Geometry check sheet. Reference: the model listing, model coordinates, mm. A direction names the side the tool comes from. Coordinates: 2 decimals unless noted, no trailing zeros. Write each loop counter-clockwise with the first axis right and the second up, starting at its lowest first coordinate (ties: lowest second). Pieces come first, ordered by that corner, then holes. Notation, with made-up numbers: (6, 36.25) -> (55, 36.25) arc R16 ccw to (55, 46.25) -> close; hole circle Ø8 at (39.25, 38.5). An arc over 180 degrees is marked (long way). One line per question, with ' | ' between items.
```python
from build123d import *

# Parameters (mm, degrees)
SKETCH1_R           = 5
BOSS_EXTRUDE1_DEPTH = 5
FILLET1_R           = 5
SKETCH2_R           = 0.6
CUT_EXTRUDE1_DEPTH  = 5
SKETCH3_R           = 0.6
CUT_EXTRUDE2_DEPTH  = 2.5
BOSS_EXTRUDE7_REACH = 72.882
BOSS_EXTRUDE8_DEPTH = 35
SKETCH13_R          = 1
SKETCH13_W          = 14
SKETCH13_H          = 24
CUT_EXTRUDE3_DEPTH  = 82.57977968
SKETCH14_W          = 10
SKETCH14_H          = 35
BOSS_EXTRUDE9_DEPTH = 5
SKETCH15_R          = 1.25
CUT_EXTRUDE4_DEPTH  = 5
SKETCH16_R          = 1.25
CUT_EXTRUDE5_DEPTH  = 96.984672029
FILLET2_R           = 5


with BuildPart() as part:
    # Sketch1 → Boss-Extrude1 (new body)
    with BuildSketch(Plane.XY):
        with BuildLine():
            ThreePointArc((0, 10), (-10, 0), (0, -10))
            ThreePointArc((0, -10), (30, -5.393920142), (60, -10))
            ThreePointArc((60, -10), (70, 0), (60, 10))
            ThreePointArc((60, 10), (30, 5.393920142), (0, 10))
        make_face()
        Circle(SKETCH1_R, mode=Mode.SUBTRACT)
        with Locations((60, 0)):
            Circle(SKETCH1_R, mode=Mode.SUBTRACT)
    extrude(amount=BOSS_EXTRUDE1_DEPTH)

    # Fillet1
    fillet1_edges = [part.edges().sort_by_distance(p)[0] for p in [
        (60, 10, 2.5),
        (60, -10, 2.5),
        (0, -10, 2.5),
        (0, 10, 2.5),
    ]]
    fillet(fillet1_edges, radius=FILLET1_R)

    # Sketch2 → Cut-Extrude1 (cut)
    with BuildSketch(Plane(origin=(0, 0, 0), x_dir=(-1, 0, 0), z_dir=(0, 0, -1))):
        with Locations((-4.45, 0)):
            Circle(SKETCH2_R)
        with Locations((-6.45, 0)):
            Circle(SKETCH2_R)
        with Locations((-8.45, 0)):
            Circle(SKETCH2_R)
        with Locations((-10.45, 0)):
            Circle(SKETCH2_R)
        with Locations((-12.45, 0)):
            Circle(SKETCH2_R)
        with Locations((-14.45, 0)):
            Circle(SKETCH2_R)
    cut_extrude1 = extrude(amount=-CUT_EXTRUDE1_DEPTH, mode=Mode.SUBTRACT)

    # Sketch3 → Cut-Extrude2 (cut)
    with BuildSketch(Plane(origin=(0, 0, 0), x_dir=(-1, 0, 0), z_dir=(0, 0, -1))):
        with BuildLine():
            Line((-15.012283737, -2.435946838), (-1.124567474, -4.871893677))
            ThreePointArc((-1.124567474, -4.871893677), (-3.832599709, -3.211102532), (-4.993539326, -0.254096441))
            ThreePointArc((-4.993539326, -0.254096441), (-5.05, 0), (-4.993539326, 0.254096441))
            ThreePointArc((-4.993539326, 0.254096441), (-3.746221254, 3.311468906), (-0.865051903, 4.924600005))
            Line((-0.865051903, 4.924600005), (-14.882525952, 2.462300002))
            ThreePointArc((-14.882525952, 2.462300002), (-16.949123268, 0.066203422), (-15.012283737, -2.435946838))
        make_face()
        with Locations((-12.45, 0)):
            Circle(SKETCH3_R, mode=Mode.SUBTRACT)
        with Locations((-6.45, 0)):
            Circle(SKETCH3_R, mode=Mode.SUBTRACT)
        with Locations((-8.45, 0)):
            Circle(SKETCH3_R, mode=Mode.SUBTRACT)
        with Locations((-10.45, 0)):
            Circle(SKETCH3_R, mode=Mode.SUBTRACT)
        with Locations((-14.45, 0)):
            Circle(SKETCH3_R, mode=Mode.SUBTRACT)
    cut_extrude2 = extrude(amount=-CUT_EXTRUDE2_DEPTH, mode=Mode.SUBTRACT)

    # Mirror2: Cut-Extrude1, Cut-Extrude2 across plane
    add(cut_extrude1.mirror(Plane(origin=(30, 0, 0), x_dir=(0, 0, 1), z_dir=(1, 0, 0))), mode=Mode.SUBTRACT)
    add(cut_extrude2.mirror(Plane(origin=(30, 0, 0), x_dir=(0, 0, 1), z_dir=(1, 0, 0))), mode=Mode.SUBTRACT)

    # Boss-Extrude7: up to this face of the body (flat: up to its plane)
    boss_extrude7_end = Plane(part.part.faces().sort_by_distance((30, 0, 5))[0])
    # Sketch11 → Boss-Extrude7 (add, up to the picked face)
    with BuildSketch(Plane(origin=(0, 0, 0), x_dir=(-1, 0, 0), z_dir=(0, 0, -1)), mode=Mode.PRIVATE) as boss_extrude7_sk1:
        with BuildLine():
            ThreePointArc((-14.882525952, 2.462300002), (-16.949123268, 0.066203422), (-15.012283737, -2.435946838))
            Line((-15.012283737, -2.435946838), (0, -5))
            ThreePointArc((0, -5), (4.981114334, 0.434165854), (-0.865051903, 4.924600005))
            Line((-0.865051903, 4.924600005), (-14.882525952, 2.462300002))
        make_face()
    boss_extrude7_tool1 = split(extrude(boss_extrude7_sk1.sketch, amount=-BOSS_EXTRUDE7_REACH, mode=Mode.PRIVATE), bisect_by=boss_extrude7_end, keep=Keep.BOTH, mode=Mode.PRIVATE)
    add(boss_extrude7_tool1.solids().sort_by(Axis((4.874327, 0.014975, 0), (0, 0, 1)))[0])

    # Sketch12 → Boss-Extrude8 (add)
    with BuildSketch(Plane.XY.offset(5)):
        with BuildLine():
            ThreePointArc((-9.682458366, 2.5), (-10, 0), (-9.682458366, -2.5))
            Line((-9.682458366, -2.5), (10.317541634, -2.5))
            Line((10.317541634, -2.5), (10.317541634, 2.5))
            Line((10.317541634, 2.5), (-9.682458366, 2.5))
        make_face()
    extrude(amount=BOSS_EXTRUDE8_DEPTH)

    # Sketch13 → Cut-Extrude3 (cut, through all)
    with BuildSketch(Plane(origin=(0, 2.5, 0), x_dir=(1, 0, 0), z_dir=(0, 1, 0))):
        with Locations(Location((0.317541634, -8.6, 0), (0, 0, 270))):
            Circle(SKETCH13_R)
        with Locations(Location((0.317541634, -36.4, 0), (0, 0, 270))):
            Circle(SKETCH13_R)
        with Locations((0.317541634, -22.5)):
            Rectangle(SKETCH13_W, SKETCH13_H)
    extrude(amount=-CUT_EXTRUDE3_DEPTH, mode=Mode.SUBTRACT)

    # Sketch14 → Boss-Extrude9 (add)
    with BuildSketch(Plane(origin=(0, 2.5, 0), x_dir=(1, 0, 0), z_dir=(0, 1, 0))):
        with Locations((-11.682458366, -22.5)):
            Rectangle(SKETCH14_W, SKETCH14_H)
    extrude(amount=-BOSS_EXTRUDE9_DEPTH)

    # Sketch15 → Cut-Extrude4 (cut)
    with BuildSketch(Plane(origin=(0, 2.5, 0), x_dir=(1, 0, 0), z_dir=(0, 1, 0))):
        with Locations(Location((-11.682458366, -22.5, 0), (0, 0, 270))):
            Circle(SKETCH15_R)
    extrude(amount=-CUT_EXTRUDE4_DEPTH, mode=Mode.SUBTRACT)

    # Sketch16 → Cut-Extrude5 (cut, through all)
    with BuildSketch(Plane.ZY.offset(16.682458366)):
        with Locations((22.5, 0)):
            Circle(SKETCH16_R)
    extrude(amount=-CUT_EXTRUDE5_DEPTH, mode=Mode.SUBTRACT)

    # Fillet2
    fillet2_edges = [part.edges().sort_by_distance(p)[0] for p in [
        (10.317541634, 0, 40),
        (-16.682458366, 0, 5),
        (-16.682458366, 0, 40),
    ]]
    fillet(fillet2_edges, radius=FILLET2_R)


solid = part.part
```
(1) Tool access check on faces 5 (the face through (-9, 2.5, 22)), 6 (the face through (51.834, -3.637, 1.232)), 7 (the face through (10.318, 0, 20)). Record the directions out of +Z, -Z, +X, -X, +Y, -Y that give a thin tool (end or side, any length) a straight path to the whole face; none if there is none.
Answers below:
face 5: +Z, +X, -X, +Y | face 6: -Z | face 7: +Z, +X, +Y, -Y
(2) Cross-section at A-A (z = 33.5). Record the cut outline in (x, y).
Answers below:
outline: (-16.68, -2.5) -> (-6.68, -2.5) -> (-6.68, 2.5) -> (-16.68, 2.5) -> close; (7.32, -2.5) -> (10.32, -2.5) -> (10.32, 2.5) -> (7.32, 2.5) -> close
(3) Cross-section at C-C (y = -7.75). Record the cut outline in (x, z).
Answers below:
outline: (-6.32, 0) -> (8.42, 0) -> (8.42, 5) -> (-6.32, 5) -> close; (51.58, 0) -> (66.32, 0) -> (66.32, 5) -> (51.58, 5) -> close
(4) Cross-section at B-B (z = 22.5). Record the cut outline in (x, y), plus the area to 4 significant figures.
Answers below:
outline: (-16.68, -2.5) -> (-12.93, -2.5) -> (-12.93, -1.25) -> (-16.68, -1.25) -> close; (-16.68, 1.25) -> (-12.93, 1.25) -> (-12.93, 2.5) -> (-16.68, 2.5) -> close; (-10.43, -2.5) -> (-6.68, -2.5) -> (-6.68, -1.25) -> (-10.43, -1.25) -> close; (-10.43, 1.25) -> (-6.68, 1.25) -> (-6.68, 2.5) -> (-10.43, 2.5) -> close; (7.32, -2.5) -> (10.32, -2.5) -> (10.32, -1.25) -> (7.32, -1.25) -> close; (7.32, 1.25) -> (10.32, 1.25) -> (10.32, 2.5) -> (7.32, 2.5) -> close | area: 26.25 mm²
(5) Draft check along Y on faces 1 (the face through (51, -1, 2.5)), 2 (the face through (52.22, 3.71, 1.23)), 3 (the face through (29.586, -5.395, 2.465)), 4 (the face through (-6.682, 2, 23)). Enter one of: pulls with the +Y half, pulls with the -Y half, needs draft (parallel to the pull), parting line crosses it, or undercut.
Answers below:
face 1: undercut | face 2: undercut | face 3: pulls with the -Y half | face 4: needs draft
(6) Material ranges on line 1 (X direction, y = -0.75, z = 20); line 2 (Z direction, x = 49.5, y = 1); line 3 (Z direction, x = 58.5, y = -7), recorded low to high.
Answers below:
line 1: x = -16.68 to -6.68, 7.32 to 10.32 | line 2: z = 2.5 to 5 | line 3: z = 0 to 5
(7) Cross-section at D-D (x = -5.5). Record the cut outline in (y, z).
Answers below:
outline: (-8.35, 0) -> (8.35, 0) -> (8.35, 5) -> (2.5, 5) -> (2.5, 10.5) -> (-2.5, 10.5) -> (-2.5, 5) -> (-8.35, 5) -> close; (-2.5, 34.5) -> (2.5, 34.5) -> (2.5, 40) -> (-2.5, 40) -> close
(8) Depth check by flat-ended pin: P1, Ø0.6, axis at x = -11, y = -0.5, coming from the -Z side; P2, Ø4, axis at x = -11.68, z = 22.5, coming from the +Y side; P3, Ø2, axis at x = 26, y = 5.5, coming from the +Z side. Enter the tip coordinate at first touch or a pass-through.
Answers below:
P1: stops at z = 5 | P2: stops at y = 2.5 | P3: stops at z = 5
